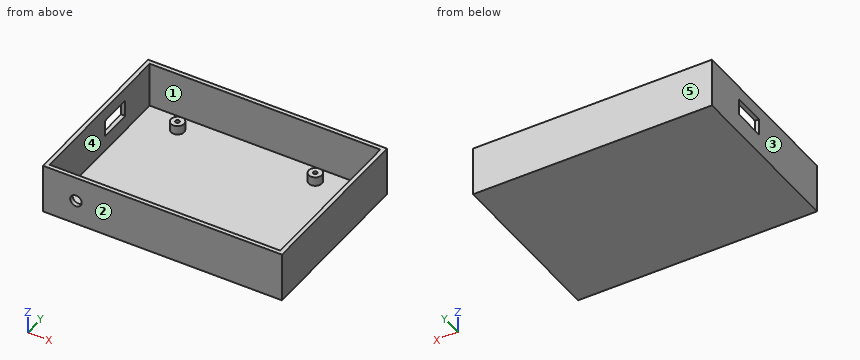
```python
from build123d import *

# Parameters (mm, degrees)
SKETCH_W        = 145
SKETCH_H        = 105
PAD_DEPTH       = 30
SKETCH002_W     = 140
SKETCH002_H     = 100
POCKET_DEPTH    = 27.5
SKETCH003_R     = 4
SKETCH003_R_2   = 1
PAD001_DEPTH    = 5.5
SKETCH004_W     = 20
SKETCH004_H     = 10
POCKET001_DEPTH = 2.5
SKETCH005_R     = 3.5
POCKET002_DEPTH = 2.5
SKETCH006_R     = 1.25
POCKET003_DEPTH = 7.5


with BuildPart() as part:
    # Sketch → Pad (new body)
    with BuildSketch(Plane.XY):
        with Locations((72.5, 52.5)):
            Rectangle(SKETCH_W, SKETCH_H)
    extrude(amount=PAD_DEPTH)

    # Sketch002 (on Face6 of Pad) → Pocket (cut)
    with BuildSketch(Plane.XY.offset(30)):
        with Locations((72.5, 52.5)):
            Rectangle(SKETCH002_W, SKETCH002_H)
    extrude(amount=-POCKET_DEPTH, mode=Mode.SUBTRACT)

    # Sketch003 (on Face11 of Pocket) → Pad001 (join)
    with BuildSketch(Plane.XY.offset(2.5)):
        with Locations((25.5, 92.5)):
            Circle(SKETCH003_R)
        with Locations((25.5, 92.5)):
            Circle(SKETCH003_R_2, mode=Mode.SUBTRACT)
        with Locations((109.08, 92.5)):
            Circle(SKETCH003_R)
        with Locations((109.08, 92.5)):
            Circle(SKETCH003_R_2, mode=Mode.SUBTRACT)
        with Locations((25.5, 18.7)):
            Circle(SKETCH003_R)
        with Locations((25.5, 18.7)):
            Circle(SKETCH003_R_2, mode=Mode.SUBTRACT)
        with Locations((130.7, 8.5)):
            Circle(SKETCH003_R)
        with Locations((130.7, 8.5)):
            Circle(SKETCH003_R_2, mode=Mode.SUBTRACT)
    extrude(amount=PAD001_DEPTH)

    # Sketch004 (on Face2 of Pad001) → Pocket001 (cut)
    with BuildSketch(Plane(origin=(0, 0, 0), x_dir=(0, -1, 0), z_dir=(-1, 0, 0))):
        with Locations((-68, 17)):
            Rectangle(SKETCH004_W, SKETCH004_H)
    extrude(amount=-POCKET001_DEPTH, mode=Mode.SUBTRACT)

    # Sketch005 (on Face1 of Pocket001) → Pocket002 (cut)
    with BuildSketch(Plane.XZ):
        with Locations((20, 15)):
            Circle(SKETCH005_R)
    extrude(amount=-POCKET002_DEPTH, mode=Mode.SUBTRACT)

    # Sketch006 (on Face21 of Pocket002) → Pocket003 (cut)
    with BuildSketch(Plane.XY.offset(8)):
        with Locations((25.5, 92.5)):
            Circle(SKETCH006_R)
        with Locations((109.08, 92.5)):
            Circle(SKETCH006_R)
        with Locations((25.5, 18.7)):
            Circle(SKETCH006_R)
        with Locations((130.7, 8.5)):
            Circle(SKETCH006_R)
    extrude(amount=-POCKET003_DEPTH, mode=Mode.SUBTRACT)


solid = part.part
```
Geometry check sheet. Reference: the model listing, model coordinates, mm. Face numbers are marked on the shaded views. A direction names the side the tool comes from. Give positions to 0.01 mm unless a question says otherwise; leave off trailing zeros. Order: outer loops, then holes, each group sorted by start corner. A loop starts at its lowest first (then second) coordinate and runs counter-clockwise, first axis right, second up.
1. Access from +Z, -Z, +X, -X, +Y, -Y to the whole of each face (thin tool, end or side, straight path). Record for the marked faces 1 and 2.
2. Section check B-B, the plane x = 20. Enter the section's corners in (y, z), and give its area (4 significant figures).
3. Section check D-D, the plane z = 25.5. Enter the section's corners in (x, y).
4. Section check C-C, the plane y = 79.5. Enter the section's corners in (x, z), and give its area (3 significant figures).
5. Gauge pin test, flat ends, axial feed: pin 1 Ø3 at (x, y) = (109.08, 92.5) entering from +Z; pin 2 Ø0.8 at (x, y) = (25, 18.5) entering from +Z; pin 3 Ø3 at (x, y) = (87, 86.5) entering from +Z. Record the tip position at first contact, or that the pin passes through.
6. Section check A-A, the plane z = 4.25. Give the number of separate pieces and of enclosed holes in the cut face, and give its area (3 significant figures).
7. Thickness scan on L1, parallel to X at y = 38.5, z = 15.5; L2, parallel to Y at x = 80, z = 17.5; L3, parallel to Z at x = 20, y = 1.95. Record the ranges inside material, lowest first.
8. Release check for a two-part mould opening along Y. For the marked faces 3, 4 and 5 record: pulls with the +Y half, pulls with the -Y half, needs draft (parallel to the pull), parting line crosses it, or undercut.
Values follow:
1. face 1: +Z
1. face 2: +Z, -Z, +X, -X, -Y
2. outline: (0, 0) - (105, 0) - (105, 30) - (102.5, 30) - (102.5, 2.5) - (2.5, 2.5) - (2.5, 11.5) - (0, 11.5) - close; (0, 18.5) - (2.5, 18.5) - (2.5, 30) - (0, 30) - close
2. area: 382.5 mm2
3. outline: (0, 0) - (145, 0) - (145, 105) - (0, 105) - close; hole (2.5, 2.5) - (142.5, 2.5) - (142.5, 102.5) - (2.5, 102.5) - close
4. outline: (0, 0) - (145, 0) - (145, 30) - (142.5, 30) - (142.5, 2.5) - (2.5, 2.5) - (2.5, 30) - (0, 30) - close
4. area: 500 mm2
5. pin 1: stops at z = 8
5. pin 2: stops at z = 0.5
5. pin 3: stops at z = 2.5
6. separate pieces: 5
6. enclosed holes: 5
6. area: 1,410 mm2
7. L1: x = 0 to 2.5, 142.5 to 145
7. L2: y = 0 to 2.5, 102.5 to 105
7. L3: z = 0 to 11.5, 18.5 to 30
8. face 3: needs draft
8. face 4: undercut
8. face 5: pulls with the +Y half
